Geometry: see drawing. Coordinates: mm, zero at the bounding-box minimum. Coordinates: 2 decimals unless noted, no trailing zeros. Loops run counter-clockwise (first coordinate to the right, second up) from the corner with the lowest first, then second, coordinate; pieces in that order, holes last. Notation, with made-up numbers: (56, 22.5) - (73, 22.5) arc R12 ccw to (73, 41.5) - close; hole circle Ø4 at (64, 42). An arc over 180 degrees is marked (long way). Use one line per item in the form item = value.
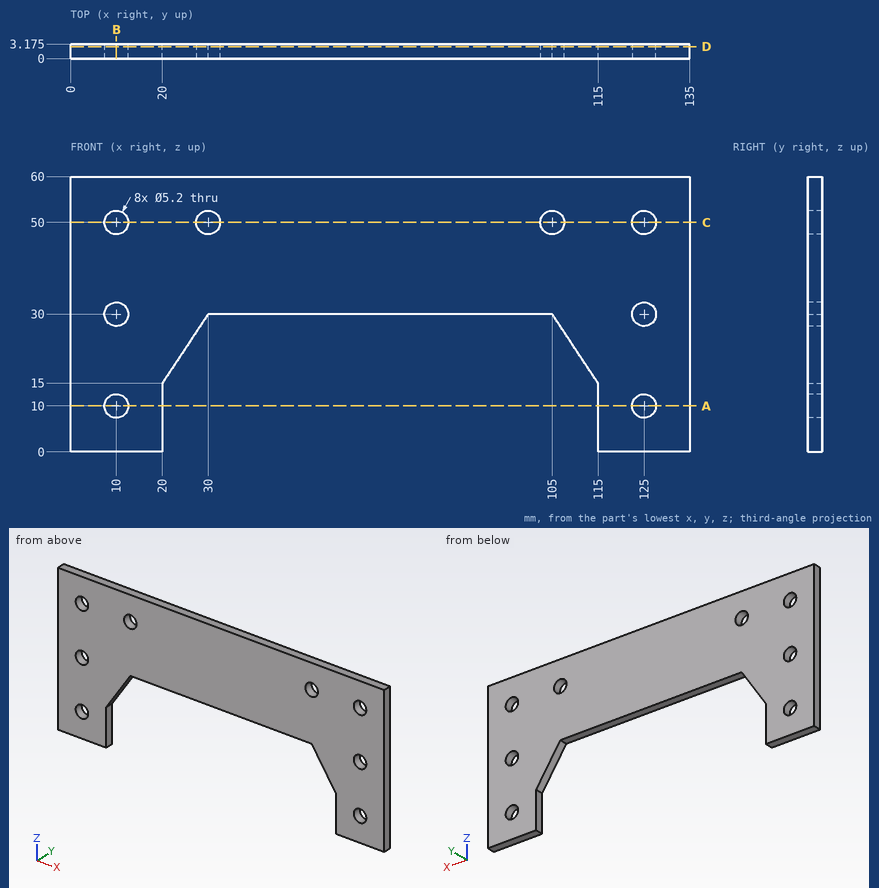
Q1. Cut plane C-C, the plane z = 50. Return loops of the section in (x, y) (3 decimals).
Check values:
outline = (0, 0) - (7.4, 0) - (7.4, 3.175) - (0, 3.175) - close; (12.6, 0) - (27.4, 0) - (27.4, 3.175) - (12.6, 3.175) - close; (32.6, 0) - (102.4, 0) - (102.4, 3.175) - (32.6, 3.175) - close; (107.6, 0) - (122.4, 0) - (122.4, 3.175) - (107.6, 3.175) - close; (127.6, 0) - (135, 0) - (135, 3.175) - (127.6, 3.175) - close
Q2. Cut plane B-B, the plane x = 10. Return loops of the section in (y, z) (3 decimals).
Check values:
outline = (0, 0) - (3.175, 0) - (3.175, 7.4) - (0, 7.4) - close; (0, 12.6) - (3.175, 12.6) - (3.175, 27.4) - (0, 27.4) - close; (0, 32.6) - (3.175, 32.6) - (3.175, 47.4) - (0, 47.4) - close; (0, 52.6) - (3.175, 52.6) - (3.175, 60) - (0, 60) - close
Q3. First-contact query: P1, Ø7, axis at x = 125, z = 10, coming from the +Y side (3 decimals); P2, Ø4.5, axis at x = 125, z = 30, coming from the -Y side; P3, Ø1, axis at x = 97.5, y = 0.5, coming from the -Z side. Flat tips, straight axial feed; report the tip coordinate or a pass-through.
Check values:
P1 = 3.175
P2 = through
P3 = 30
Q4. Cut plane A-A, the plane z = 10. Return loops of the section in (x, y) (3 decimals), then the cut area to 3 significant figures.
Check values:
outline = (0, 0) - (7.4, 0) - (7.4, 3.175) - (0, 3.175) - close; (12.6, 0) - (20, 0) - (20, 3.175) - (12.6, 3.175) - close; (115, 0) - (122.4, 0) - (122.4, 3.175) - (115, 3.175) - close; (127.6, 0) - (135, 0) - (135, 3.175) - (127.6, 3.175) - close
area = 94.0 mm²
Q5. Cut plane D-D, the plane y = 2.6. Give the number of separate pieces and of enclosed holes in the cut face, then the cut area to 3 significant figures.
Check values:
separate_pieces = 1
enclosed_holes = 8
area = 5,230 mm²
Q6. Ray query, line 1 along Z through (x, y) = (10, 2.4); line 2 along X through (y, z) = (1.85, 50); line 3 along X through (y, z) = (0.95, 10). Return the intervals inside material, ascending. Write a range as [from, to].
Check values:
line_1 = [0, 7.4], [12.6, 27.4], [32.6, 47.4], [52.6, 60]
line_2 = [0, 7.4], [12.6, 27.4], [32.6, 102.4], [107.6, 122.4], [127.6, 135]
line_3 = [0, 7.4], [12.6, 20], [115, 122.4], [127.6, 135]
